Geometry check sheet. Reference: the model listing, model coordinates, mm. Face numbers are marked on the shaded views. Round coordinates to 2 decimals unless told otherwise and drop trailing zeros. Write each loop counter-clockwise with the first axis right and the second up, starting at its lowest first coordinate (ties: lowest second). Pieces come first, ordered by that corner, then holes. Notation, with made-up numbers: M 23.25,13 L 41.25,13 A32 ccw 41.25,40 Z; hole C -6,13 d6. An arc over 180 degrees is marked long. Answer in a Markdown table with one row per item. Add a question column.
from build123d import *

# Parameters (mm, degrees)
EXTRUDE_1_DEPTH      = 30
SKETCH_2_R           = 44.45
CUT_EXTRUDE_1_DEPTH  = 4
SKETCH_3_R           = 25.5
SKETCH_3_R_2         = 2.25
CUT_EXTRUDE_2_DEPTH  = 188.619295383
CUT_EXTRUDE_3_DEPTH  = 189.215302247
SKETCH_5_R           = 1.65
CUT_EXTRUDE_4_DEPTH  = 189.215302247
EXTRUDE_START        = -30
EXTRUDE_2_DEPTH      = 30
CUT_EXTRUDE_5_DEPTH  = 198.040604952
CUT_EXTRUDE_7_DEPTH  = 233.432785983
CUT_EXTRUDE_8_DEPTH  = 233.432785983
CUT_EXTRUDE_9_DEPTH  = 233.432785983
FILLET_1_R           = 5
CUT_EXTRUDE_10_DEPTH = 233.432785983
EXTRUDE_START_2      = -5
EXTRUDE_3_DEPTH      = 5
EXTRUDE_4_DEPTH      = 5
SKETCH_14_R          = 4.25
CUT_EXTRUDE_11_DEPTH = 189.364728478
SKETCH_16_W          = 43
SKETCH_16_H          = 30
CUT_EXTRUDE_12_DEPTH = 233.432785983
EXTRUDE_7_REACH      = 188.592
SKETCH_18_W          = 210
SKETCH_18_H          = 5
EXTRUDE_8_DEPTH      = 210
EXTRUDE_9_DEPTH      = 5
EXTRUDE_10_DEPTH     = 5
SKETCH_22_R          = 4.25
CUT_EXTRUDE_13_DEPTH = 187.984035343
FILLET_2_R           = 5
CUT_EXTRUDE_14_DEPTH = 234.418610938


with BuildPart() as part:
    # 草图1 → 凸台-拉伸1 (new body)
    with BuildSketch(Plane(origin=(0, 0, 0), x_dir=(1, 0, 0), z_dir=(0, 1, 0))):
        with BuildLine():
            Line((170, 31.93), (170, -31.93))
            ThreePointArc((170, -31.93), (167.781993847, -38.210172909), (162.111885646, -41.704453387))
            Line((162.111885646, -41.704453387), (15.839142344, -73.308400404))
            ThreePointArc((15.839142344, -73.308400404), (-75, 0), (15.839142344, 73.308400404))
            Line((15.839142344, 73.308400404), (162.111885646, 41.704453387))
            ThreePointArc((162.111885646, 41.704453387), (167.781993847, 38.210172909), (170, 31.93))
        make_face()
    extrude(amount=EXTRUDE_1_DEPTH)

    # 草图2 → 切除-拉伸1 (cut)
    with BuildSketch(Plane(origin=(0, 30, 0), x_dir=(1, 0, 0), z_dir=(0, 1, 0))):
        with Locations(Location((0, 0, 0), (0, 0, 270))):
            Circle(SKETCH_2_R)
    extrude(amount=-CUT_EXTRUDE_1_DEPTH, mode=Mode.SUBTRACT)

    # 草图3 → 切除-拉伸2 (cut, through all)
    with BuildSketch(Plane(origin=(0, 26, 0), x_dir=(1, 0, 0), z_dir=(0, 1, 0))):
        with Locations(Location((0, 0, 0), (0, 0, 270))):
            Circle(SKETCH_3_R)
        with Locations(Location((0, 41, 0), (0, 0, 270))):
            Circle(SKETCH_3_R_2)
        with Locations(Location((28.991378029, 28.991378029, 0), (0, 0, 270))):
            Circle(SKETCH_3_R_2)
        with Locations(Location((41, 0, 0), (0, 0, 270))):
            Circle(SKETCH_3_R_2)
        with Locations(Location((28.991378029, -28.991378029, 0), (0, 0, 270))):
            Circle(SKETCH_3_R_2)
        with Locations(Location((0, -41, 0), (0, 0, 270))):
            Circle(SKETCH_3_R_2)
        with Locations(Location((-28.991378029, -28.991378029, 0), (0, 0, 270))):
            Circle(SKETCH_3_R_2)
        with Locations(Location((-41, 0, 0), (0, 0, 270))):
            Circle(SKETCH_3_R_2)
        with Locations(Location((-28.991378029, 28.991378029, 0), (0, 0, 270))):
            Circle(SKETCH_3_R_2)
    extrude(amount=-CUT_EXTRUDE_2_DEPTH, mode=Mode.SUBTRACT)

    # 草图4 → 切除-拉伸3 (cut, through all)
    with BuildSketch(Plane(origin=(0, 30, 0), x_dir=(1, 0, 0), z_dir=(0, 1, 0))):
        with BuildLine():
            Line((124, 18.5), (134, 18.5))
            ThreePointArc((134, 18.5), (152.5, 0), (134, -18.5))
            Line((134, -18.5), (124, -18.5))
            ThreePointArc((124, -18.5), (105.5, 0), (124, 18.5))
        make_face()
    extrude(amount=-CUT_EXTRUDE_3_DEPTH, mode=Mode.SUBTRACT)

    # 草图5 → 切除-拉伸4 (cut, through all)
    with BuildSketch(Plane(origin=(0, 30, 0), x_dir=(1, 0, 0), z_dir=(0, 1, 0))):
        with Locations(Location((116.75, 25.5, 0), (0, 0, 270))):
            Circle(SKETCH_5_R)
        with Locations(Location((141.25, 25.5, 0), (0, 0, 270))):
            Circle(SKETCH_5_R)
        with Locations(Location((141.25, -25.5, 0), (0, 0, 270))):
            Circle(SKETCH_5_R)
        with Locations(Location((116.75, -25.5, 0), (0, 0, 270))):
            Circle(SKETCH_5_R)
    extrude(amount=-CUT_EXTRUDE_4_DEPTH, mode=Mode.SUBTRACT)

    # 草图6 → 凸台-拉伸2 (add)
    with BuildSketch(Plane(origin=(0, 30, 0), x_dir=(1, 0, 0), z_dir=(0, 1, 0)).offset(EXTRUDE_START)):
        with BuildLine():
            Line((158, 95), (-52, 95))
            Line((-52, 95), (-52, 54.046276467))
            ThreePointArc((-52, 54.046276467), (-20.48558667, 72.148047366), (15.839142344, 73.308400404))
            Line((15.839142344, 73.308400404), (158, 42.592874655))
            Line((158, 42.592874655), (158, 95))
        make_face()
        with BuildLine():
            ThreePointArc((15.839142344, -73.308400404), (-20.48558667, -72.148047366), (-52, -54.046276467))
            Line((-52, -54.046276467), (-52, -95))
            Line((-52, -95), (158, -95))
            Line((158, -95), (158, -42.592874655))
            Line((158, -42.592874655), (15.839142344, -73.308400404))
        make_face()
    extrude(amount=EXTRUDE_2_DEPTH)

    # 草图7 → 切除-拉伸5 (cut, through all)
    with BuildSketch(Plane(origin=(0, 30, 0), x_dir=(1, 0, 0), z_dir=(0, 1, 0))):
        with BuildLine():
            Line((-52, 54.046276467), (-52, -54.046276467))
            ThreePointArc((-52, -54.046276467), (-75, 0), (-52, 54.046276467))
        make_face()
        with BuildLine():
            Line((158, 42.592874655), (158, -42.592874655))
            Line((158, -42.592874655), (162.111885646, -41.704453387))
            ThreePointArc((162.111885646, -41.704453387), (167.781993847, -38.210172909), (170, -31.93))
            Line((170, -31.93), (170, 31.93))
            ThreePointArc((170, 31.93), (167.781993847, 38.210172909), (162.111885646, 41.704453387))
            Line((162.111885646, 41.704453387), (158, 42.592874655))
        make_face()
    extrude(amount=-CUT_EXTRUDE_5_DEPTH, mode=Mode.SUBTRACT)

    # 草图9 → 切除-拉伸7 (cut, through all)
    with BuildSketch(Plane.ZY.offset(52)):
        Polygon((-95, 20), (-60, 10.621778265), (-60, 30), (-95, 30), align=None)
    extrude(amount=-CUT_EXTRUDE_7_DEPTH, mode=Mode.SUBTRACT)

    # 草图10 → 切除-拉伸8 (cut, through all)
    with BuildSketch(Plane.ZY.offset(52)):
        Polygon((-95, 12.753066737), (-52, 1.231251463), (-52, 0), (-95, 0), align=None)
    extrude(amount=-CUT_EXTRUDE_8_DEPTH, mode=Mode.SUBTRACT)

    # 草图8 → 切除-拉伸9 (cut, through all)
    with BuildSketch(Plane.ZY.offset(52)):
        Polygon((0, 0), (52, 0), (52, 17.3), (-52, 17.3), (-52, 0), align=None)
    extrude(amount=-CUT_EXTRUDE_9_DEPTH, mode=Mode.SUBTRACT)

    # 圆角1
    fillet_1_edges = [part.edges().sort_by_distance(p)[0] for p in [
        (53, 10.621778265, -60),
    ]]
    fillet(fillet_1_edges, radius=FILLET_1_R)

    # 草图11 → 切除-拉伸10 (cut, through all)
    with BuildSketch(Plane.ZY.offset(52)):
        Polygon((-95, 12.753066737), (-93.188266684, 19.514547521), (-95, 20), align=None)
    extrude(amount=-CUT_EXTRUDE_10_DEPTH, mode=Mode.SUBTRACT)

    # 草图12 → 凸台-拉伸3 (add)
    with BuildSketch(Plane.ZY.offset(52).offset(EXTRUDE_START_2)):
        with BuildLine():
            Line((-93.188266684, 19.514547521), (-60, 30))
            Line((-60, 30), (-60, 17.137905129))
            ThreePointArc((-60, 17.137905129), (-61.956192855, 13.171138428), (-66.294095226, 12.308275998))
            Line((-66.294095226, 12.308275998), (-93.188266684, 19.514547521))
        make_face()
    extrude(amount=EXTRUDE_3_DEPTH)

    # 草图13 → 凸台-拉伸4 (add)
    with BuildSketch(Plane(origin=(158, 0, 0), x_dir=(0, 0, -1), z_dir=(1, 0, 0))):
        with BuildLine():
            Line((66.294095226, 12.308275998), (93.188266684, 19.514547521))
            Line((93.188266684, 19.514547521), (60, 30))
            Line((60, 30), (60, 17.137905129))
            ThreePointArc((60, 17.137905129), (61.956192855, 13.171138428), (66.294095226, 12.308275998))
        make_face()
    extrude(amount=-EXTRUDE_4_DEPTH)

    # 草图14 → 切除-拉伸11 (cut, through all)
    with BuildSketch(Plane(origin=(0, -5.089745962, -1.36379332), x_dir=(1, 0, 0), z_dir=(0, 0.9659258262890681, 0.2588190451025214))):
        with Locations(Location((-27, 82.063690052, 0), (0, 0, 270))):
            Circle(SKETCH_14_R)
        with Locations(Location((23, 82.063690052, 0), (0, 0, 270))):
            Circle(SKETCH_14_R)
        with Locations(Location((83, 82.063690052, 0), (0, 0, 270))):
            Circle(SKETCH_14_R)
        with Locations(Location((133, 82.063690052, 0), (0, 0, 270))):
            Circle(SKETCH_14_R)
    extrude(amount=-CUT_EXTRUDE_11_DEPTH, mode=Mode.SUBTRACT)

    # 草图16 → 切除-拉伸12 (cut, through all)
    with BuildSketch(Plane.ZY.offset(52)):
        with Locations((73.5, 15)):
            Rectangle(SKETCH_16_W, SKETCH_16_H)
    extrude(amount=-CUT_EXTRUDE_12_DEPTH, mode=Mode.SUBTRACT)

    # 凸台-拉伸7: up to this plane
    extrude_7_end = Plane(origin=(0, -11.851226746, -3.175526636), z_dir=(0, -0.9659258262890681, -0.25881904510252146))
    # 草图18 → 凸台-拉伸7 (add, up to the surface)
    with BuildSketch(Plane(origin=(0, 30, 0), x_dir=(1, 0, 0), z_dir=(0, 1, 0)), mode=Mode.PRIVATE) as extrude_7_sk1:
        with Locations((53, -54.5)):
            Rectangle(SKETCH_18_W, SKETCH_18_H)
    extrude_7_tool1 = split(extrude(extrude_7_sk1.sketch, amount=-EXTRUDE_7_REACH, mode=Mode.PRIVATE), bisect_by=extrude_7_end, keep=Keep.BOTH, mode=Mode.PRIVATE)
    add(extrude_7_tool1.solids().sort_by_distance((53, 30, 54.5))[0])

    # 草图19 → 凸台-拉伸8 (add)
    with BuildSketch(Plane.ZY.offset(52)):
        Polygon((57, -27.975210512), (90.188266684, -36.867979769), (92, -30.106498985), (57, -20.72827725), align=None)
    extrude(amount=-EXTRUDE_8_DEPTH)

    # 草图20 → 凸台-拉伸9 (add)
    with BuildSketch(Plane.ZY.offset(52)):
        Polygon((92, -30.106498985), (57, -20.72827725), (57, 30), align=None)
    extrude(amount=-EXTRUDE_9_DEPTH)

    # 草图21 → 凸台-拉伸10 (add)
    with BuildSketch(Plane(origin=(158, 0, 0), x_dir=(0, 0, -1), z_dir=(1, 0, 0))):
        Polygon((-57, 30), (-92, -30.106498985), (-57, -20.72827725), align=None)
    extrude(amount=-EXTRUDE_10_DEPTH)

    # 草图22 → 切除-拉伸13 (cut, through all)
    with BuildSketch(Plane(origin=(0, -5.089745962, -1.36379332), x_dir=(1, 0, 0), z_dir=(0, 0.9659258262890686, 0.25881904510251946))):
        with Locations(Location((-27, -77.936309948, 0), (0, 0, 270))):
            Circle(SKETCH_22_R)
        with Locations(Location((23, -69.936309948, 0), (0, 0, 270))):
            Circle(SKETCH_22_R)
        with Locations(Location((83, -69.936309948, 0), (0, 0, 270))):
            Circle(SKETCH_22_R)
        with Locations(Location((133, -77.936309948, 0), (0, 0, 270))):
            Circle(SKETCH_22_R)
    extrude(amount=-CUT_EXTRUDE_13_DEPTH, mode=Mode.SUBTRACT)

    # 圆角2
    fillet_2_edges = [part.edges().sort_by_distance(p)[0] for p in [
        (53, -20.72827725, 57),
    ]]
    fillet(fillet_2_edges, radius=FILLET_2_R)

    # 草图23 → 切除-拉伸14 (cut, through all)
    with BuildSketch(Plane.ZY.offset(52)):
        Polygon((-52, 17.3), (-52, 40.52409207), (98.672945053, 40.52409207), (98.672945053, -43.91232927), (-52, -43.91232927), align=None)
    extrude(amount=-CUT_EXTRUDE_14_DEPTH, mode=Mode.SUBTRACT)


solid = part.part
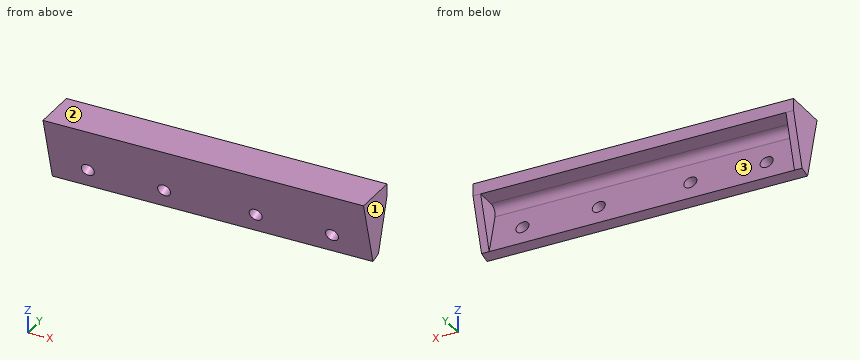
Item 1: Gauge pin test, flat end, axial feed: pin 1 Ø6.5 at (x, y) = (47.5, 23) entering from -Z. Record the tip position at first contact, or that the pin passes through.
Item 2: Section check B-B, the plane y = 28.25. Record the boundary of the cut face in (x, z), and give its area (3 significant figures).
Item 3: Section check D-D, the plane x = 131. Record the boundary of the cut face in (y, z), and give its area (3 significant figures).
Item 4: Section check A-A, the plane x = -3. Record the boundary of the cut face in (y, z).
Item 5: Section check C-C, the plane z = -74. Record the boundary of the cut face in (x, y), and give its area (3 significant figures).
Item 6: Mould release check, pull along Z, two halves, no side actions. Record for the marked faces 1, 2 and 3: +Z half, -Z half, draft (parallel to the pull), parting line (faces both ways), or undercut.
Item 7: Scan lines: probe 1 along X at (y, z) = (12.5, -64); probe 2 along Z at (x, y) = (-34, 26.75); probe 3 along X at (y, z) = (10.75, -78.5). Record each from-to range of solid material in increasing order. Write a range as from..to.
Result sheet:
| question | item | result |
|---|---|---|
| 1 | pin 1 | stops at z = -60 |
| 2 | outline | M -52,-65.54 L -47,-65.54 L -47,-60 L 153,-60 L 153,-65.54 L 158,-65.54 L 158,-52 L -52,-52 Z |
| 2 | area | 1,740 mm^2 |
| 3 | outline | M 1.23,-52 L 8.42,-78.82 L 15.18,-77.01 L 12.31,-66.29 A5 cw 17.14,-60 L 30,-60 L 30,-52 Z; M 10.36,-86.07 L 12.75,-95 L 19.51,-93.19 L 17.12,-84.25 Z |
| 3 | area | 426 mm^2 |
| 4 | outline | M 1.23,-52 L 12.75,-95 L 19.51,-93.19 L 12.31,-66.29 A5 cw 17.14,-60 L 30,-60 L 30,-52 Z |
| 5 | outline | M -52,7.13 L 158,7.13 L 158,25.58 L 153,25.58 L 153,14.37 L -47,14.37 L -47,25.58 L -52,25.58 Z |
| 5 | area | 1,630 mm^2 |
| 6 | face 1 | draft |
| 6 | face 2 | +Z half |
| 6 | face 3 | undercut |
| 7 | probe 1 | x = -52..-47, 153..158 |
| 7 | probe 2 | z = -60..-52 |
| 7 | probe 3 | x = -52..-29.47, -24.53..20.53, 25.47..80.53, 85.47..130.53, 135.47..158 |
